For this review, take the finished solid that the model builds, in its own axes (mm). Round coordinates to 2 decimals unless told otherwise and drop trailing zeros. Write each loop counter-clockwise with the first axis right and the second up, starting at its lowest first coordinate (ties: lowest second). Pieces come first, ordered by that corner, then holes. Notation, with made-up numbers: (10, 74) -> (28, 74) arc R27 cw to (28, 94) -> close; hole circle Ø6 at (-35, 70). An arc over 180 degrees is marked (long way). Answer as CSV lines item,"result". Start each with the question number.
Item 1: Take a section at B-B on x = 0. Give the boundary of the cut face in (y, z) (3 decimals).
Item 2: Wall thickness on probe 1 along X at (y, z) = (2.95, 0) (3 decimals); probe 2 along Y at (x, z) = (-0.5, 2.25); probe 3 along X at (y, z) = (83, -3.75): over which ranges is each line inside the solid? List them lowest first. Write a range as from..to.
Item 3: Take a section at C-C on y = 12. Give the boundary of the cut face in (x, z).
Item 4: For pin 1 Ø3 at (x, z) = (-0.5, -0.5) entering from +Y; pin 2 Ø5 at (x, z) = (0, 0) entering from -Y, all flat-tipped, find the tip position at first contact; note any pin that passes through.
Item 5: Take a section at A-A on z = 0. Give the boundary of the cut face in (x, y) (3 decimals), then the cut area to 3 significant figures.
```python
from build123d import *

# Parameters (mm, degrees)
SKETCH1_W           = 10
SKETCH1_H           = 10
BOSS_EXTRUDE1_DEPTH = 160
FILLET1_R           = 3
SKETCH2_R           = 3.125
CUT_EXTRUDE1_DEPTH  = 4.7
CUT_EXTRUDE2_START  = -160
SKETCH2_2_R         = 3.125
CUT_EXTRUDE2_DEPTH  = 4.7


with BuildPart() as part:
    # Sketch1 → Boss-Extrude1 (new body)
    with BuildSketch(Plane(origin=(0, 0, 0), x_dir=(1, 0, 0), z_dir=(0, 1, 0))):
        Rectangle(SKETCH1_W, SKETCH1_H)
    extrude(amount=BOSS_EXTRUDE1_DEPTH)

    # Fillet1
    fillet1_edges = [part.edges().sort_by_distance(p)[0] for p in [
        (-5, 80, -5),
        (5, 80, -5),
        (5, 80, 5),
        (-5, 80, 5),
    ]]
    fillet(fillet1_edges, radius=FILLET1_R)

    # Sketch2 → Cut-Extrude1 (cut)
    with BuildSketch(Plane(origin=(0, 160, 0), x_dir=(1, 0, 0), z_dir=(0, 1, 0))):
        with Locations(Location((0, 0, 0), (0, 0, 270))):
            Circle(SKETCH2_R)
    extrude(amount=-CUT_EXTRUDE1_DEPTH, mode=Mode.SUBTRACT)

    # Sketch2<2> → Cut-Extrude2 (cut)
    with BuildSketch(Plane(origin=(0, 160, 0), x_dir=(1, 0, 0), z_dir=(0, 1, 0)).offset(CUT_EXTRUDE2_START)):
        with Locations(Location((0, 0, 0), (0, 0, 270))):
            Circle(SKETCH2_2_R)
    extrude(amount=CUT_EXTRUDE2_DEPTH, mode=Mode.SUBTRACT)


solid = part.part
```
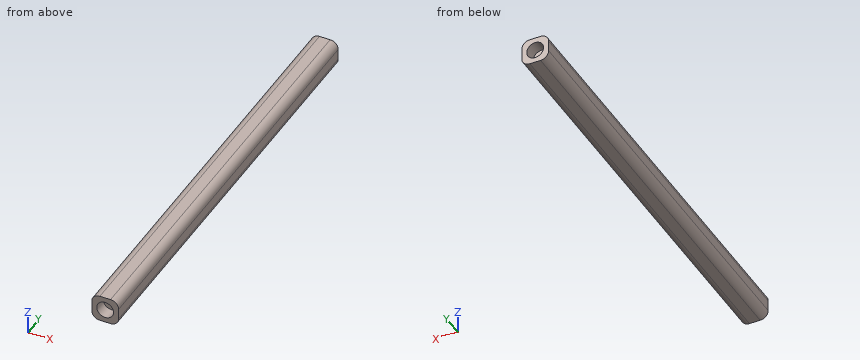
Output values:
1,outline,"(0, -5) -> (160, -5) -> (160, -3.125) -> (155.3, -3.125) -> (155.3, 3.125) -> (160, 3.125) -> (160, 5) -> (0, 5) -> (0, 3.125) -> (4.7, 3.125) -> (4.7, -3.125) -> (0, -3.125) -> close"
2,probe 1,"x = -5..-3.125, 3.125..5"
2,probe 2,"y = 4.7..155.3"
2,probe 3,"x = -4.44..4.44"
3,outline,"(-5, -2) arc R3 ccw to (-2, -5) -> (2, -5) arc R3 ccw to (5, -2) -> (5, 2) arc R3 ccw to (2, 5) -> (-2, 5) arc R3 ccw to (-5, 2) -> close"
4,pin 1,"stops at y = 155.3"
4,pin 2,"stops at y = 4.7"
5,outline,"(-5, 0) -> (-3.125, 0) -> (-3.125, 4.7) -> (3.125, 4.7) -> (3.125, 0) -> (5, 0) -> (5, 160) -> (3.125, 160) -> (3.125, 155.3) -> (-3.125, 155.3) -> (-3.125, 160) -> (-5, 160) -> close"
5,area,"1,540 mm^2"
